Print and shaded views of the part. All mm, measured from the part's lowest x, y and z. A direction names the side the tool comes from. Round coordinates to 2 decimals unless told otherwise and drop trailing zeros. Write each loop counter-clockwise with the first axis right and the second up, starting at its lowest first coordinate (ties: lowest second). Pieces come first, ordered by that corner, then holes. Notation, with made-up numbers: (2.25, 73.25) - (21.25, 73.25) arc R9 ccw to (21.25, 90.25) - close; hole circle Ø9 at (81, 23.25). An arc over 180 degrees is marked (long way). Put each result on its own line as item: value. Start each with the question number.
Item 1: Cut at C-C (z = 86.5). Give the cut face in (x, y).
Item 2: Mould opens along Z. For the marked faces 3, 4, 5 and 6 say: released by +Z, released by -Z, zero draft, split by the parting line, or undercut.
Item 3: 3-axis set-ups, long thin cutter, end or side, ignore diameter. For the marked faces 1 and 2: which of +Z, -Z, +X, -X, +Y, -Y reach the whole face in a straight line?
Item 4: Cut at B-B (y = 29). Give the cut face in (x, z), and give its area (3 significant figures).
Item 5: Drill centre lines: line 1 (Z direction, x = 10.5, y = 23.5) (1 decimal); line 2 (Z direction, x = 83.5, y = 46) (1 decimal); line 3 (X direction, y = 14.5, z = 15) (1 decimal). Where is each one in solid material? Low to high. Write a range as from..to.
Item 6: Cut at A-A (x = 13). Give the cut face in (y, z), and give its area (3 significant figures).
Item 7: Pin check, flat tip, straight feed: pin 1 Ø15.5 at (x, z) = (17.16, 20.74) entering from -Y. Stop position of the tip, or through.
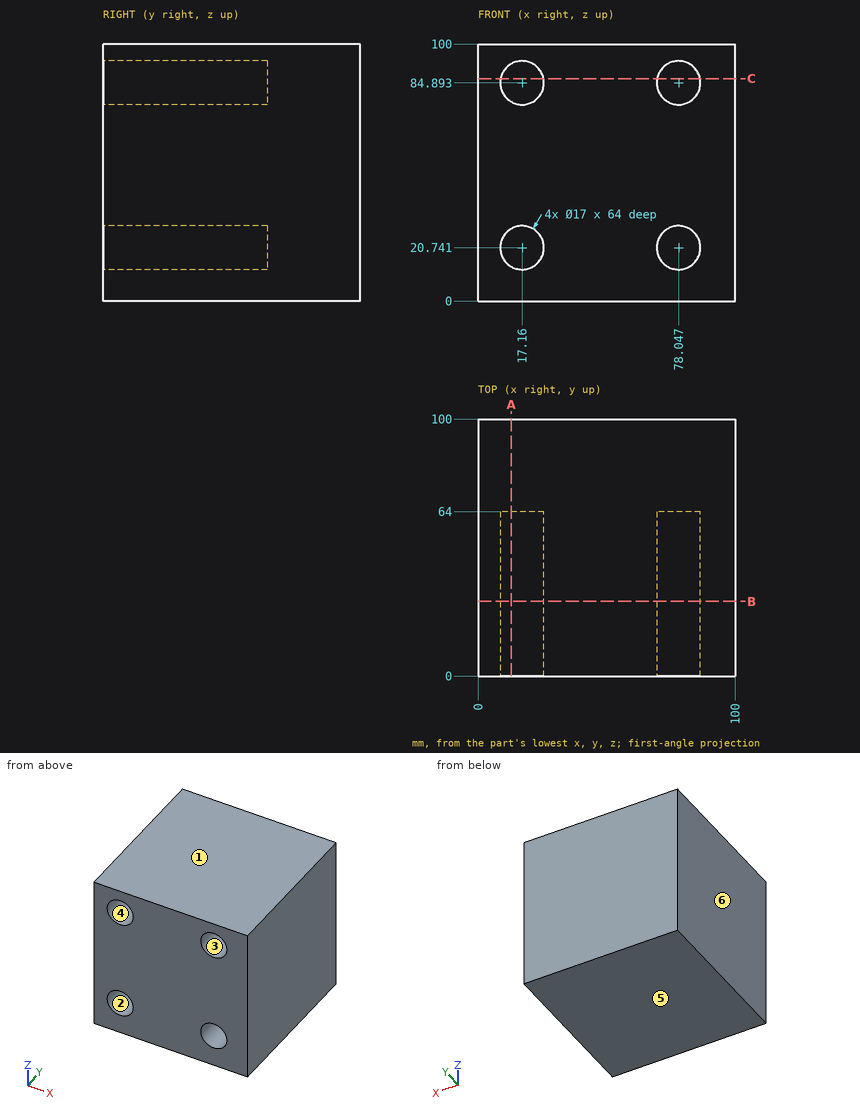
Output values:
1. outline: (0, 0) - (8.81, 0) - (8.81, 64) - (25.51, 64) - (25.51, 0) - (69.7, 0) - (69.7, 64) - (86.39, 64) - (86.39, 0) - (100, 0) - (100, 100) - (0, 100) - close
2. face 3: undercut
2. face 4: undercut
2. face 5: released by -Z
2. face 6: zero draft
3. face 1: +Z, +X, -X, +Y, -Y
3. face 2: -Y
4. outline: (0, 0) - (100, 0) - (100, 100) - (0, 100) - close; hole circle Ø17 at (17.16, 20.74); hole circle Ø17 at (17.16, 84.89); hole circle Ø17 at (78.05, 20.74); hole circle Ø17 at (78.05, 84.89)
4. area: 9,090 mm2
5. line 1: 0..15.5, 26..79.6, 90.2..100
5. line 2: 0..14.2, 27.3..78.4, 91.4..100
5. line 3: 0..10.9, 23.4..71.8, 84.3..100
6. outline: (0, 0) - (100, 0) - (100, 100) - (0, 100) - (0, 92.31) - (64, 92.31) - (64, 77.48) - (0, 77.48) - (0, 28.15) - (64, 28.15) - (64, 13.33) - (0, 13.33) - close
6. area: 8,100 mm2
7. pin 1: y = 64
